Could you check a few things on this model? Use its own coordinates, in mm. A direction names the side the tool comes from. Coordinates: 2 decimals unless noted, no trailing zeros. Order: outer loops, then holes, each group sorted by start corner. A loop starts at its lowest first (then second) coordinate and runs counter-clockwise, first axis right, second up. Notation, with made-up numbers: (40, -35.5) - (49, -35.5) arc R29 cw to (49, -9.5) - close; hole circle Ø1 at (-39, 57). An arc over 180 degrees is marked (long way). Answer as a JSON object with one key per item and string values. Group by question number.
(1) Imagine slicing it at A-A, the plane y = 0. Write out the boundary of the cut face in (x, z), and give its area (3 significant figures).
(2) Will these pins go through, and if not, where does the flat tip stop? P1, Ø4, axis at y = -6, z = 24, coming from the -X side; P2, Ø9.5, axis at x = 41.5, y = 41.5, coming from the -Z side; P3, Ø1, axis at y = -4, z = 19, coming from the +X side; P4, Ø1.5, axis at x = 11, z = 29, coming from the +Y side.
(3) Please list where these lines run through material, in increasing order: probe 1 along X at (y, z) = (-41, 7); probe 2 along X at (y, z) = (-47, 9).
(4) Imagine slicing it at C-C, the plane y = -41.5. Write out the boundary of the cut face in (x, z), and give its area (3 significant figures).
(5) Which directions (+Z, -Z, +X, -X, +Y, -Y) give clear straight access to the entire face, cutting with the end or side of a thin tool? Please do faces 1 (the flat face through (-35, 24, 14)), 2 (the flat face through (1, -54, 6)).
Autodesk Inventor part; units mm, degrees
ref_plane "YZ Plane" through (0, 0, 0) normal (1, 0, 0) x (0, 1, 0)
ref_plane "XZ Plane" through (0, 0, 0) normal (0, 1, 0) x (-1, 0, 0)
ref_plane "XY Plane" through (0, 0, 0) normal (0, 0, 1) x (1, 0, 0)
sketch "Sketch1" plane through (0, 0, 0) normal (0, 0, 1) x (1, 0, 0)
  line L0 (-54, 54) -> (54, 54)
  line L1 (54, 54) -> (54, -54)
  line L2 (54, -54) -> (-54, -54)
  line L3 (-54, -54) -> (-54, 54)
  line L4 (-54, 54) -> (54, -54) construction
  line L5 (54, 54) -> (-54, -54) construction
  point P0 (0, 0)
  dimension "d0" = 108
extrude "Extrusion1" add sketch "Sketch1" along normal blind 14
sketch "Sketch2" plane through (0, 0, 14) normal (0, 0, 1) x (1, 0, 0)
  circle A0 centre (-41.5, 41.5) radius 6
  line L0 (54, 54) -> (-54, 54) construction
  line L1 (-54, 54) -> (0, 0) construction
  dimension "d4" = 41.5
  dimension "d5" = 12
extrude "Extrusion2" cut sketch "Sketch2" against normal through all
pattern_circular "Circular Pattern1" count 4 over 360 about axis through (0, 0, -10) along (0, 0, 1) of "Extrusion2"
fillet "Fillet1" radius 10 4 edges at (-54, 54, 7) (54, 54, 7) (-54, -54, 7) (54, -54, 7)
sketch "Sketch4" plane through (0, 0, 0) normal (0, 0, 1) x (1, 0, 0)
  circle A0 centre (0, 0) radius 35
  dimension "d15" = 70
extrude "Extrusion4" add sketch "Sketch4" along normal blind 31
sketch "Sketch5" plane through (0, 0, 0) normal (0, 0, 1) x (1, 0, 0)
  circle A0 centre (0, 0) radius 15
  dimension "d18" = 30
extrude "Extrusion5" cut sketch "Sketch5" along normal blind 31
sketch "Sketch6" plane through (0, 0, 0) normal (0, 0, 1) x (1, 0, 0)
  circle A0 centre (0, 0) radius 15
  circle A1 centre (0, 0) radius 21
  dimension "d21" = 6
extrude "Extrusion6" add sketch "Sketch6" along normal blind 40
fillet "Fillet2" radius 3 2 edges at (-35, 0, 31) (-35, 0, 14)
fillet "Fillet3" radius 2 8 edges at (-51.0711, 51.0711, 14) (-54, 0, 14) (-51.0711, -51.0711, 14) (0, -54, 14) (51.0711, -51.0711, 14) (54, 0, 14) (51.0711, 51.0711, 14) (0, 54, 14)
properties part number "NDM-VOS dummy Disc Harrow Pillow block bearing mount Assembly"
Result set:
{
 "1": {"outline": "(-54, 0) - (-15, 0) - (-15, 40) - (-21, 40) - (-21, 31) - (-32, 31) arc R3 ccw to (-35, 28) - (-35, 17) arc R3 cw to (-38, 14) - (-52, 14) arc R2 ccw to (-54, 12) - close; (15, 0) - (54, 0) - (54, 12) arc R2 ccw to (52, 14) - (38, 14) arc R3 cw to (35, 17) - (35, 28) arc R3 ccw to (32, 31) - (21, 31) - (21, 40) - (15, 40) - close", "area": "1,880 mm^2"},
 "2": {"P1": "stops at x = -34.77", "P2": "passes through", "P3": "stops at x = 34.82", "P4": "stops at y = 33.37"},
 "3": {"probe 1": "x = -54 to -47.48, -35.52 to 35.52, 47.48 to 54", "probe 2": "x = -53.54 to -43.9, -39.1 to 39.1, 43.9 to 53.54"},
 "4": {"outline": "(-54, 0) - (-47.5, 0) - (-47.5, 14) - (-52, 14) arc R2 ccw to (-54, 12) - close; (-35.5, 0) - (35.5, 0) - (35.5, 14) - (-35.5, 14) - close; (47.5, 0) - (54, 0) - (54, 12) arc R2 ccw to (52, 14) - (47.5, 14) - close", "area": "1,170 mm^2"},
 "5": {"face 1": "+Z", "face 2": "+Z, -Z, +X, -X, -Y"}
}
